Autodesk Inventor part; units mm, degrees
ref_plane "YZ Plane" through (0, 0, 0) normal (1, 0, 0) x (0, 1, 0)
ref_plane "XZ Plane" through (0, 0, 0) normal (0, 1, 0) x (-1, 0, 0)
ref_plane "XY Plane" through (0, 0, 0) normal (0, 0, 1) x (1, 0, 0)
sketch "Sketch1" plane through (0, 0, 0) normal (0, 0, 1) x (1, 0, 0)
  line L0 (0, 0) -> (0, 59.721302)
  line L1 (60.981972, 120.067993) -> (120.7, 119.442605)
  arc A0 (60.981972, 120.067993) -> (0, 59.721302) centre (60.35, 59.721302) ccw
  dimension "d0" = 120.7
  dimension "d1" = 120.7
  dimension "d2" = 60.35
  dimension "d7" = 89.4
sketch "Sketch2" plane through (0, 0, 0) normal (0, 1, 0) x (-1, 0, 0)
  circle A0 centre (0, 0) radius 25.4
  circle A1 centre (0, 0) radius 23.75
  dimension "d4" = 1.65
  dimension "d5" = 50.8
sweep "Sweep1" add profiles "Sketch2" path "Sketch1"
equation "\"d1\" = d0"
equation "\"d2\" = 0.5 * d0"
properties part number "ASME BPE - 89.4 DEG Elbow-50.8"
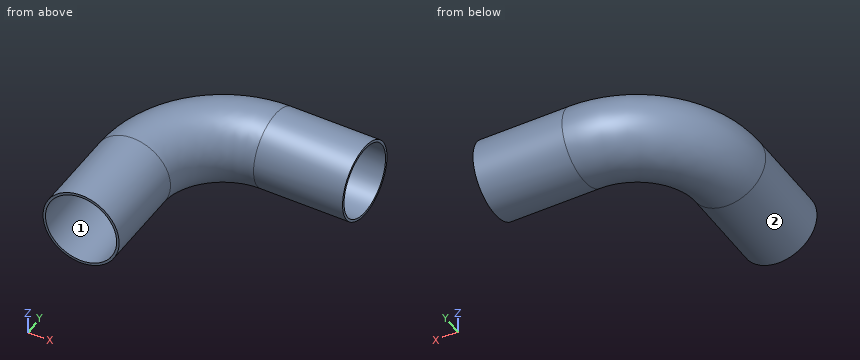
Model file for the job. Use its own axes, mm. Face numbers are marked on the shaded views. Give positions to 0.01 mm unless a question says otherwise; leave off trailing zeros. Loops run counter-clockwise (first coordinate to the right, second up) from the corner with the lowest first, then second, coordinate; pieces in that order, holes last.
1) Flat gauge pins, fed straight in: pin 1 Ø1 at (x, y) = (20.5, 100.5) entering from -Z; pin 2 Ø3 at (x, z) = (70, 9) entering from -Y; pin 3 Ø6 at (x, y) = (16, 44.5) entering from -Z. Where does each tip first touch, or does it go through?
2) Wall check: line 1 (Z direction, x = 0, y = 20); line 2 (Y direction, x = 47, z = -17); line 3 (X direction, y = 26.5, z = 21.5). Give the ranges that are in metal, low to high.
3) Pull direction X, two halves, no side cores. Call the marked faces 1 and 2: +X half, -X half, draft (parallel to the pull), parting line (faces both ways), or undercut.
4) Saw through at A-A (y = 51). Write the cut outline in (x, z), plus the area to 3 significant figures.
Answer block:
1. pin 1: stops at z = -25.24
1. pin 2: stops at y = 95.7
1. pin 3: stops at z = -21.82
2. line 1: z = -25.4 to -23.75, 23.75 to 25.4
2. line 2: y = 98.99 to 101.4, 135.49 to 137.81
2. line 3: x = -13.52 to -10.09, 10.09 to 13.52
3. face 1: undercut
3. face 2: parting line
4. outline: circle Ø50.8 at (0, 0); hole circle Ø47.5 at (0, 0)
4. area: 255 mm2
